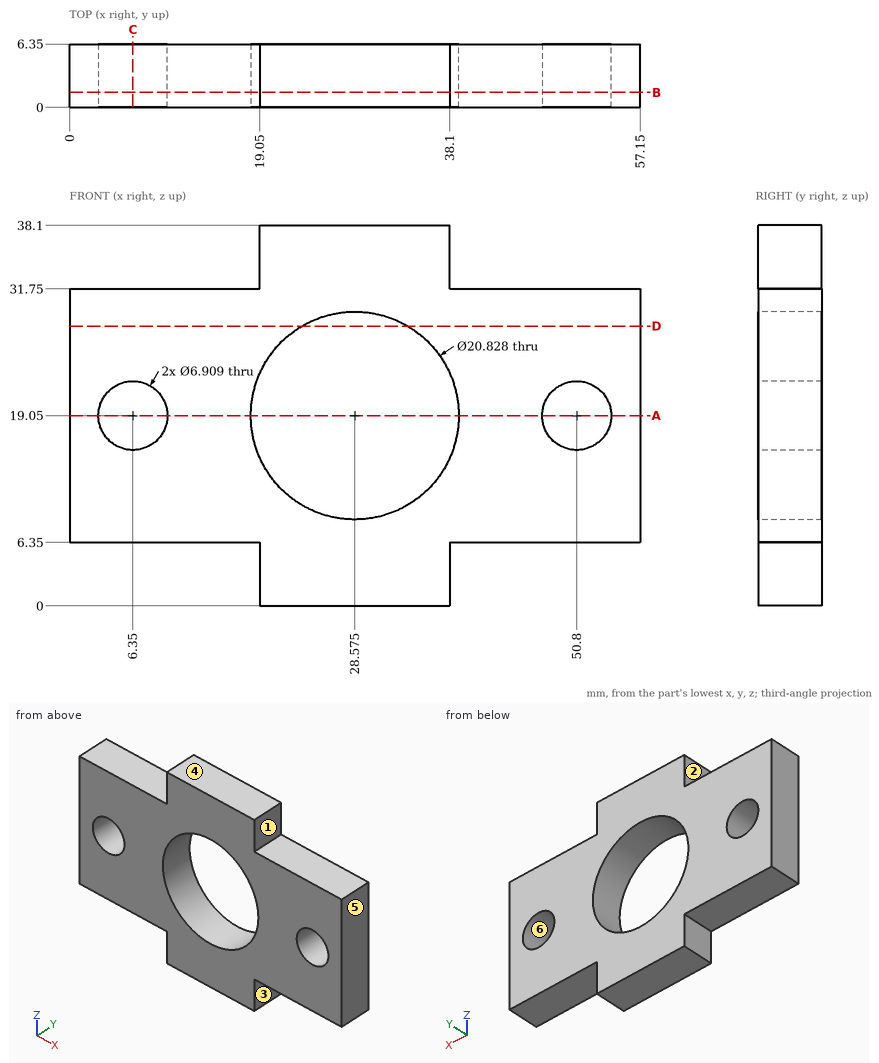
Study the drawing (mm; zero at the part's minimum x, y, z) and answer. A direction names the side the tool comes from. Round coordinates to 2 decimals unless told otherwise and drop trailing zeros. Write each loop counter-clockwise with the first axis right and the second up, starting at its lowest first coordinate (ties: lowest second). Pieces come first, ordered by that corner, then holes. Notation, with made-up numbers: (63, -9.75) -> (97, -9.75) arc R15 ccw to (97, 11.25) -> close; hole circle Ø5 at (84.5, 14.5). An arc over 180 degrees is marked (long way). Use CSV: the item, a comma, the result in double quotes. Start each with the question number.
(1) Section A-A on z = 19.05 is taken. Give the vertices of the cut face in (x, y).
(2) Section C-C on x = 6.35 is taken. Give the vertices of the cut face in (y, z), then the cut area to 3 significant figures.
(3) Which of the six approach directions +Z, -Z, +X, -X, +Y, -Y give full straight-line access (tool end or side, diameter ignored) to the marked faces 1, 2 and 3?
(4) Consider L1, parallel to X at y = 3, z = 19.05; L2, parallel to Z at x = 15.5, y = 4.75; L3, parallel to Z at x = 5, y = 5.5. Determine where each line is inside the solid, lowest interval first. Write a range as from..to.
(5) Section B-B on y = 1.5 is taken. Count the separate pieces of the cut face and the enclosed holes in it, then the cut area to 3 significant figures.
(6) Section D-D on z = 28 is taken. Give the vertices of the cut face in (x, y), then the cut area to 3 significant figures.
(7) The mould has two halves that part along X. Classify the marked faces 4, 5 and 6: released by +X, released by -X, zero draft, split by the parting line, or undercut.
(8) Each of these flat-tipped pins is pushed along its axis until it touches: pin 1 (3 mm diameter, centred on x = 45, y = 4.5, fed in from +Z); pin 2 (1.9 mm diameter, centred on y = 4, z = 33.5, fed in from +X); pin 3 (3 mm diameter, centred on y = 4, z = 34, fed in from -X). Where does it stop, or does it pass through?
A:
1,outline,"(0, 0) -> (2.9, 0) -> (2.9, 6.35) -> (0, 6.35) -> close; (9.8, 0) -> (18.16, 0) -> (18.16, 6.35) -> (9.8, 6.35) -> close; (38.99, 0) -> (47.35, 0) -> (47.35, 6.35) -> (38.99, 6.35) -> close; (54.25, 0) -> (57.15, 0) -> (57.15, 6.35) -> (54.25, 6.35) -> close"
2,outline,"(0, 6.35) -> (6.35, 6.35) -> (6.35, 15.6) -> (0, 15.6) -> close; (0, 22.5) -> (6.35, 22.5) -> (6.35, 31.75) -> (0, 31.75) -> close"
2,area,"117 mm²"
3,face 1,"+Z, +X, +Y, -Y"
3,face 2,"+Z, -X, +Y, -Y"
3,face 3,"-Z, +X, +Y, -Y"
4,L1,"x = 0..2.9, 9.8..18.16, 38.99..47.35, 54.25..57.15"
4,L2,"z = 6.35..31.75"
4,L3,"z = 6.35..15.87, 22.23..31.75"
5,separate pieces,"1"
5,enclosed holes,"3"
5,area,"1,280 mm²"
6,outline,"(0, 0) -> (23.25, 0) -> (23.25, 6.35) -> (0, 6.35) -> close; (33.9, 0) -> (57.15, 0) -> (57.15, 6.35) -> (33.9, 6.35) -> close"
6,area,"295 mm²"
7,face 4,"zero draft"
7,face 5,"released by +X"
7,face 6,"undercut"
8,pin 1,"stops at z = 31.75"
8,pin 2,"stops at x = 38.1"
8,pin 3,"stops at x = 19.05"
